```python
from build123d import *

# Parameters (mm, degrees)
SKETCH1_R           = 101.6
BOSS_EXTRUDE1_DEPTH = 8.89
SKETCH2_R           = 25.4
CUT_EXTRUDE1_DEPTH  = 144.95885558
CUT_EXTRUDE2_DEPTH  = 144.95885558
CUT_EXTRUDE3_DEPTH  = 144.95885558
CUT_EXTRUDE10_DEPTH = 144.95885558


with BuildPart() as part:
    # Sketch1 → Boss-Extrude1 (new body)
    with BuildSketch(Plane.XY):
        Circle(SKETCH1_R)
    extrude(amount=BOSS_EXTRUDE1_DEPTH)

    # Sketch2 → Cut-Extrude1 (cut, through all)
    with BuildSketch(Plane.XY.offset(8.89)):
        Circle(SKETCH2_R)
    extrude(amount=-CUT_EXTRUDE1_DEPTH, mode=Mode.SUBTRACT)

    # Sketch3 → Cut-Extrude2 (cut, through all)
    with BuildSketch(Plane.XY.offset(8.89)):
        with BuildLine():
            ThreePointArc((69.838453591, 30.48), (0, 76.2), (-69.838453591, 30.48))
            ThreePointArc((-69.838453591, 30.48), (-63.278711326, 13.760257735), (-46.558969061, 20.32))
            ThreePointArc((-46.558969061, 20.32), (0, 50.8), (46.558969061, 20.32))
            ThreePointArc((46.558969061, 20.32), (63.278711326, 13.760257735), (69.838453591, 30.48))
        make_face()
    cut_extrude2 = extrude(amount=-CUT_EXTRUDE2_DEPTH, mode=Mode.SUBTRACT)

    # Mirror1: Cut-Extrude2 across plane
    add(cut_extrude2.mirror(Plane.ZX), mode=Mode.SUBTRACT)

    # Sketch4 → Cut-Extrude3 (cut, through all)
    with BuildSketch(Plane.XY.offset(8.89)):
        with BuildLine():
            Line((76.2, -3.175), (25.4, -3.175))
            ThreePointArc((25.4, -3.175), (22.225, 0), (25.4, 3.175))
            Line((25.4, 3.175), (76.2, 3.175))
            ThreePointArc((76.2, 3.175), (79.375, 0), (76.2, -3.175))
        make_face()
        with BuildLine():
            Line((-76.2, -3.175), (-25.4, -3.175))
            ThreePointArc((-25.4, -3.175), (-22.225, 0), (-25.4, 3.175))
            Line((-25.4, 3.175), (-76.2, 3.175))
            ThreePointArc((-76.2, 3.175), (-79.375, 0), (-76.2, -3.175))
        make_face()
    extrude(amount=-CUT_EXTRUDE3_DEPTH, mode=Mode.SUBTRACT)

    # Sketch14 → Cut-Extrude10 (cut, through all)
    with BuildSketch(Plane.XY.offset(8.89)):
        with BuildLine():
            Line((-58.198711326, -12.7), (-58.198711326, 12.7))
            ThreePointArc((-58.198711326, 12.7), (-51.242634846, 14.774417663), (-46.558969061, 20.32))
            ThreePointArc((-46.558969061, 20.32), (0, 50.8), (46.558969061, 20.32))
            ThreePointArc((46.558969061, 20.32), (51.242634846, 14.774417663), (58.198711326, 12.7))
            Line((58.198711326, 12.7), (58.198711326, -12.7))
            ThreePointArc((58.198711326, -12.7), (51.242634846, -14.774417663), (46.558969061, -20.32))
            ThreePointArc((46.558969061, -20.32), (0, -50.8), (-46.558969061, -20.32))
            ThreePointArc((-46.558969061, -20.32), (-51.242634846, -14.774417663), (-58.198711326, -12.7))
        make_face()
    extrude(amount=-CUT_EXTRUDE10_DEPTH, mode=Mode.SUBTRACT)


solid = part.part
```
Input: part model. Units: mm. Frame: model coordinates. A direction names the side the tool comes from. Coordinates: 2 decimals unless noted, no trailing zeros. Write each loop counter-clockwise with the first axis right and the second up, starting at its lowest first coordinate (ties: lowest second). Pieces come first, ordered by that corner, then holes.
1) Mould query, pull axis Y, two halves, no side actions, for faces 3 (the flat face through (60, -7, 0)), 4 (the cylindrical face through (-22.025, -99.184, 4.383)), 5 (the cylindrical face through (1.24, -76.19, 4.51)). Classes: pulls with the +Y half, pulls with the -Y half, needs draft (parallel to the pull), parting line crosses it, or undercut.
2) Pin query (flat end, axial travel): pin 1 Ø2.5 at (y, z) = (6.5, 4.5) entering from +X; pin 2 Ø5 at (y, z) = (29, 3.5) entering from +X; pin 3 Ø1 at (y, z) = (40.5, 6.5) entering from -X. Return the tip coordinate at first contact, or that it passes through.
3) Section C-C on x = 0. Output: boundary loops of the cut face in (y, z), and give its area (3 significant figures).
4) Section D-D on y = 82.5. Output: boundary loops of the cut face in (x, z).
5) Section A-A on y = 0. Output: boundary loops of the cut face in (x, z) (3 decimals), and give its area (3 significant figures).
6) Set-up query: faces 1 (the flat face through (67, -3.175, 5)), 2 (the flat face through (60, -7, 8.89)). Return all of +Z, -Z, +X, -X, +Y, -Y with unobstructed straight access to the full face (end or side cutting, diameter ignored); none if empty.
7) Section B-B on z = 2. Output: boundary loops of the cut face in (x, y) (3 decimals), and give its area (3 significant figures).
8) Material intervals for line 1 along Y through (x, z) = (60, 5.5) (3 decimals); line 2 along X through (y, z) = (-62.5, 3.25); line 3 along Y through (x, z) = (51, 1.5), sorted ascending.
Check result:
1. face 3: needs draft
1. face 4: parting line crosses it
1. face 5: undercut
2. pin 1: stops at x = 101.46
2. pin 2: stops at x = 98.08
2. pin 3: stops at x = -93.39
3. outline: (-101.6, 0) - (-76.2, 0) - (-76.2, 8.89) - (-101.6, 8.89) - close; (76.2, 0) - (101.6, 0) - (101.6, 8.89) - (76.2, 8.89) - close
3. area: 452 mm2
4. outline: (-59.3, 0) - (59.3, 0) - (59.3, 8.89) - (-59.3, 8.89) - close
5. outline: (-101.6, 0) - (-79.375, 0) - (-79.375, 8.89) - (-101.6, 8.89) - close; (79.375, 0) - (101.6, 0) - (101.6, 8.89) - (79.375, 8.89) - close
5. area: 395 mm2
6. face 1: +Z, -Z
6. face 2: +Z, +X, -X, +Y, -Y
7. outline: circle Ø203.2 at (0, 0); hole (-76.2, -3.175) - (-58.199, -3.175) - (-58.199, -12.7) arc R12.7 ccw to (-69.838, -30.48) arc R76.2 ccw to (69.838, -30.48) arc R12.7 ccw to (58.199, -12.7) - (58.199, -3.175) - (76.2, -3.175) arc R3.175 ccw to (76.2, 3.175) - (58.199, 3.175) - (58.199, 12.7) arc R12.7 ccw to (69.838, 30.48) arc R76.2 ccw to (-69.838, 30.48) arc R12.7 ccw to (-58.199, 12.7) - (-58.199, 3.175) - (-76.2, 3.175) arc R3.175 ccw to start
7. area: 15,100 mm2
8. line 1: y = -81.991 to -46.973, -12.828 to -3.175, 3.175 to 12.828, 46.973 to 81.991
8. line 2: x = -80.1 to -43.59, 43.59 to 80.1
8. line 3: y = -87.87 to -56.62, 56.62 to 87.87
